Design review of the part shown in the three views and the two pictorial views. Dimensions are in mm from the part's minimum x, y and z. Coordinates: 2 decimals unless noted, no trailing zeros. Write each loop counter-clockwise with the first axis right and the second up, starting at its lowest first coordinate (ties: lowest second). Pieces come first, ordered by that corner, then holes. Notation, with made-up numbers: M -24.5,73.25 L -19.5,73.25 A23 ccw -19.5,111.25 Z; hole C 47,76 d10. An arc over 180 degrees is marked long. One line per question, with ' | ' between items.
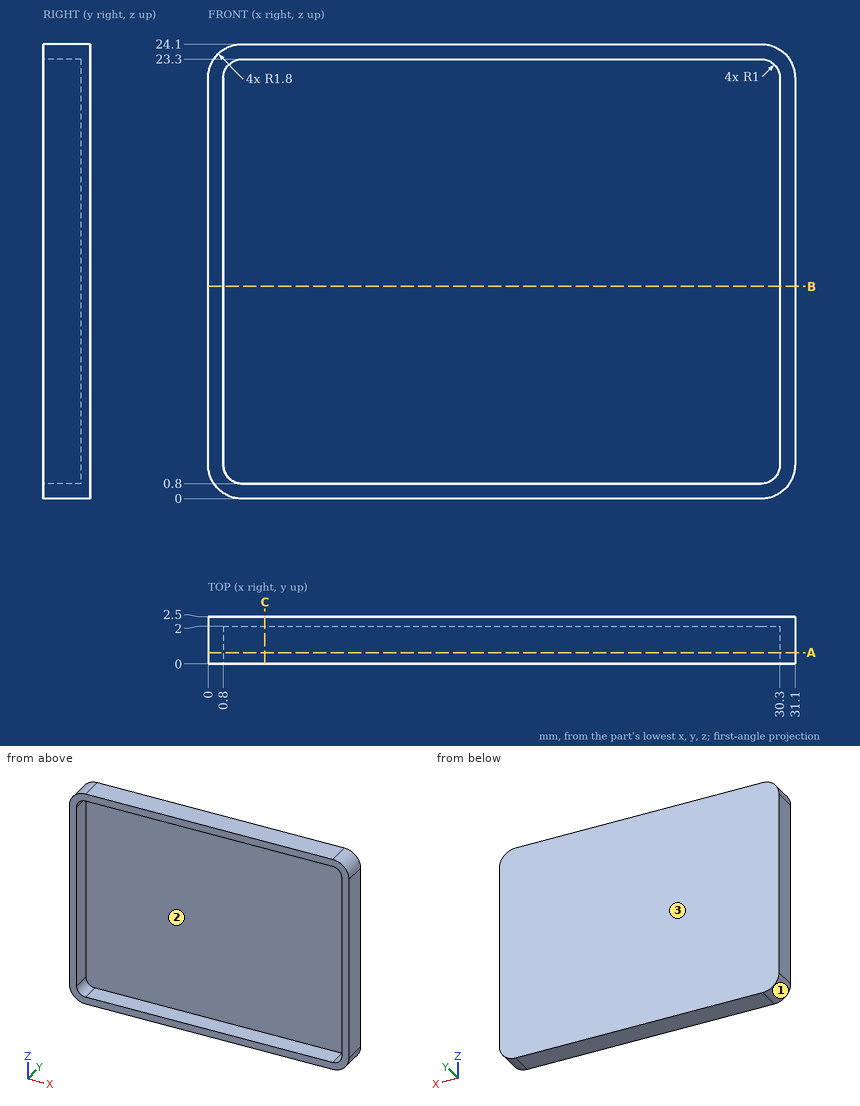
1. Take a section at C-C on x = 3. State the section outline as (y, z) points.
Computed values:
outline: M 0,0 L 2.5,0 L 2.5,24.1 L 0,24.1 L 0,23.3 L 2,23.3 L 2,0.8 L 0,0.8 Z
2. For line 1 along X through (y, z) = (0.55, 8); line 2 along Z through (x, y) = (23, 0.75); line 3 along Y through (x, z) = (3, 13.25), list the stretches that pass through material, from the lowest coordinate up.
Computed values:
line 1: x = 0 to 0.8, 30.3 to 31.1 | line 2: z = 0 to 0.8, 23.3 to 24.1 | line 3: y = 2 to 2.5
3. Clearance check with a flat-ended pin moving along its axis: P1, Ø8, axis at x = 19.5, z = 17, coming from the -Y side. State where the tip first meets the part, or that it passes through.
Computed values:
P1: stops at y = 2
4. Take a section at B-B on z = 11.25. State the section outline as (x, y) points.
Computed values:
outline: M 0,0 L 0.8,0 L 0.8,2 L 30.3,2 L 30.3,0 L 31.1,0 L 31.1,2.5 L 0,2.5 Z
5. Take a section at A-A on y = 0.6. State the section outline as (x, z) points.
Computed values:
outline: M 0,1.8 A1.8 ccw 1.8,0 L 29.3,0 A1.8 ccw 31.1,1.8 L 31.1,22.3 A1.8 ccw 29.3,24.1 L 1.8,24.1 A1.8 ccw 0,22.3 Z; hole M 0.8,1.8 A1 ccw 1.8,0.8 L 29.3,0.8 A1 ccw 30.3,1.8 L 30.3,22.3 A1 ccw 29.3,23.3 L 1.8,23.3 A1 ccw 0.8,22.3 Z
6. Draft analysis for pull direction X (two halves, no side actions). For the marked faces 1, 2 and 3, state which applies: pulls with the +X half, pulls with the -X half, needs draft (parallel to the pull), parting line crosses it, or undercut.
Computed values:
face 1: pulls with the -X half | face 2: undercut | face 3: needs draft
